Input: part model. Units: mm. Frame: model coordinates. Face numbers are marked on the shaded views. A direction names the side the tool comes from. Give positions to 0.01 mm unless a question says otherwise; leave off trailing zeros. Write each loop counter-clockwise with the first axis right and the second up, starting at its lowest first coordinate (ties: lowest second). Pieces come first, ordered by that corner, then holes. Notation, with made-up numbers: (1.25, 13.25) -> (52.25, 13.25) arc R30 cw to (52.25, 40.25) -> close; hole circle Ø2 at (48.5, 70.25). An arc over 180 degrees is marked (long way). Return JSON: item names as keys, results as strings. Group by question number.
Item 1: Section B-B, the plane x = -26. Return loops of the section in (y, z).
Item 2: Pin query (flat end, axial travel): P1, Ø2, axis at y = -16, z = 34.5, coming from the +X side. Return the tip coordinate at first contact, or that it passes through.
Item 3: Set-up query: the marked faces 1 and 2. Return all of +Z, -Z, +X, -X, +Y, -Y with unobstructed straight access to the full face (end or side cutting, diameter ignored); none if empty.
Item 4: Section C-C, the plane z = 4.5. Return loops of the section in (x, y).
Item 5: Line query: line 1 (Z direction, x = -31.5, y = -17); line 2 (Y direction, x = -10, z = -35); line 3 (X direction, y = -26.5, z = -44). Output: solid intervals per line, ascending. Write a range as [from, to].
Item 6: Mould query, pull axis Y, two halves, no side actions, for the marked faces 3, 4 and 5. Classes: released by +Y, released by -Y, zero draft, split by the parting line, or undercut.
Item 7: Section A-A, the plane y = -12.5. Return loops of the section in (x, z), then the cut area to 3 significant figures.
from build123d import *

# Parameters (mm, degrees)
F0_W     = 77.79774
F0_H     = 59.362259
F1_DEPTH = 76.2
F2_W     = 60.468386
F2_H     = 111.35032
F3_DEPTH = 50.8


with BuildPart() as f1:
    # F0 (on Right) → F1 (new body)
    with BuildSketch(Plane.YZ):
        with Locations((0, 29.681129)):
            Rectangle(F0_W, F0_H)
        with Locations((0, -29.681129)):
            Rectangle(F0_W, F0_H)
    extrude(amount=-F1_DEPTH)

    # F2 (on Right) → F3 (cut)
    with BuildSketch(Plane.YZ):
        Rectangle(F2_W, F2_H)
    extrude(amount=-F3_DEPTH, mode=Mode.SUBTRACT)


solid = f1.part
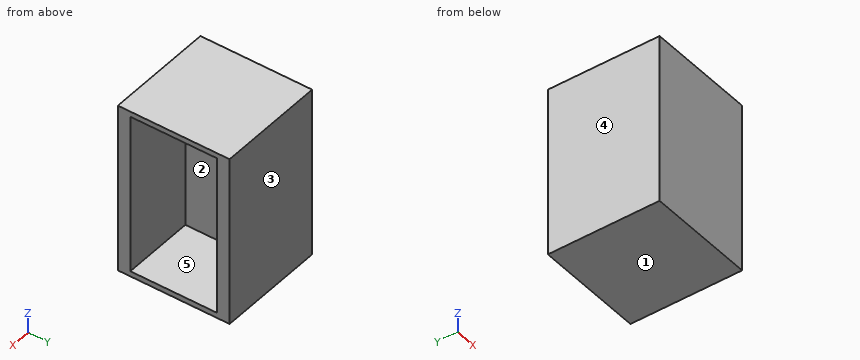
Answer below:
{
 "1": {"outline": "(-38.9, -59.36) -> (38.9, -59.36) -> (38.9, 59.36) -> (-38.9, 59.36) -> close; hole (-30.23, -55.68) -> (30.23, -55.68) -> (30.23, 55.68) -> (-30.23, 55.68) -> close"},
 "2": {"P1": "stops at x = -50.8"},
 "3": {"face 1": "-Z, +X, -X, +Y, -Y", "face 2": "+X"},
 "4": {"outline": "(-76.2, -38.9) -> (0, -38.9) -> (0, -30.23) -> (-50.8, -30.23) -> (-50.8, 30.23) -> (0, 30.23) -> (0, 38.9) -> (-76.2, 38.9) -> close"},
 "5": {"line 1": "z = [-59.36, -55.68], [55.68, 59.36]", "line 2": "y = [-38.9, -30.23], [30.23, 38.9]", "line 3": "x = [-76.2, -50.8]"},
 "6": {"face 3": "released by +Y", "face 4": "zero draft", "face 5": "undercut"},
 "7": {"outline": "(-76.2, -59.36) -> (0, -59.36) -> (0, -55.68) -> (-50.8, -55.68) -> (-50.8, 55.68) -> (0, 55.68) -> (0, 59.36) -> (-76.2, 59.36) -> close", "area": "3,390 mm2"}
}
